```python
from build123d import *

# Parameters (mm, degrees)
BOSS_EXTRUDE1_OUTLINE_R = 5.250010824
BOSS_EXTRUDE1_DEPTH     = 19
CUT_EXTRUDE1_START      = -4
SKETCH2_R               = 8.500003527
CUT_EXTRUDE1_DEPTH      = 4
SKETCH3_R               = 8.500003527
CUT_EXTRUDE2_DEPTH      = 4
CUT_EXTRUDE3_START      = -4
CUT_EXTRUDE3_DEPTH      = 4
CUT_EXTRUDE4_DEPTH      = 4


# Read off the part's stored shape, not the designer's step: Boss-Extrude1
with BuildPart() as part:
    # Boss-Extrude1 outline → Boss-Extrude1 (new body)
    with BuildSketch(Plane.XY):
        with BuildLine():
            ThreePointArc((-23.133312794, -2.201771211), (-37.271533994, 6.292181292), (-28.786231545, -7.851233083))
            Line((-28.786231545, -7.851233083), (-26.586143602, -10.066323126))
            Line((-26.586143602, -10.066323126), (-26.23976909, -10.228203619))
            ThreePointArc((-26.23976909, -10.228203619), (-24.085157131, -11.906333766), (-21.354454149, -11.947983588))
            Line((-21.354454149, -11.947983588), (-10.14791118, -7.656975592))
            Line((-10.14791118, -7.656975592), (3.746314894, -9.374802435))
            Line((3.746314894, -9.374802435), (4.037513624, -7.019745673))
            Line((4.037513624, -7.019745673), (-11.498619188, -2.842881049))
            Line((-11.498619188, -2.842881049), (-20.193931688, -5.164955939))
            Line((-20.193931688, -5.164955939), (-23.133312794, -2.201771211))
        make_face()
        with Locations((-31.26296245, 0.27993313)):
            Circle(BOSS_EXTRUDE1_OUTLINE_R, mode=Mode.SUBTRACT)
    extrude(amount=BOSS_EXTRUDE1_DEPTH)

    # Sketch2 → Cut-Extrude1 (cut)
    with BuildSketch(Plane.XY.offset(19).offset(CUT_EXTRUDE1_START)):
        with Locations((-31.26296245, 0.27993313)):
            Circle(SKETCH2_R)
    extrude(amount=CUT_EXTRUDE1_DEPTH, mode=Mode.SUBTRACT)

    # Sketch3 → Cut-Extrude2 (cut)
    with BuildSketch(Plane(origin=(0, 0, 0), x_dir=(-1, 0, 0), z_dir=(0, 0, -1))):
        with Locations((31.26296245, 0.27993313)):
            Circle(SKETCH3_R)
    extrude(amount=-CUT_EXTRUDE2_DEPTH, mode=Mode.SUBTRACT)

    # Sketch4 → Cut-Extrude3 (cut)
    with BuildSketch(Plane.XY.offset(19).offset(CUT_EXTRUDE3_START)):
        with BuildLine():
            Line((-28.786231545, -7.851233083), (-27.3768314, -9.270243736))
            ThreePointArc((-27.3768314, -9.270243736), (-23.881833101, -7.115358231), (-21.724813867, -3.621676409))
            Line((-21.724813867, -3.621676409), (-23.133312794, -2.201771211))
            ThreePointArc((-23.133312794, -2.201771211), (-25.254390905, -5.732315031), (-28.786231545, -7.851233083))
        make_face()
    extrude(amount=CUT_EXTRUDE3_DEPTH, mode=Mode.SUBTRACT)

    # Sketch5 → Cut-Extrude4 (cut)
    with BuildSketch(Plane(origin=(0, 0, 0), x_dir=(-1, 0, 0), z_dir=(0, 0, -1))):
        with BuildLine():
            Line((23.133312794, -2.201771211), (21.719099232, -3.615984773))
            ThreePointArc((21.719099232, -3.615984773), (24.169813566, -6.821498289), (27.3768314, -9.270243736))
            Line((27.3768314, -9.270243736), (28.786231545, -7.851233083))
            ThreePointArc((28.786231545, -7.851233083), (25.254390905, -5.732315031), (23.133312794, -2.201771211))
        make_face()
    extrude(amount=-CUT_EXTRUDE4_DEPTH, mode=Mode.SUBTRACT)


solid = part.part
```
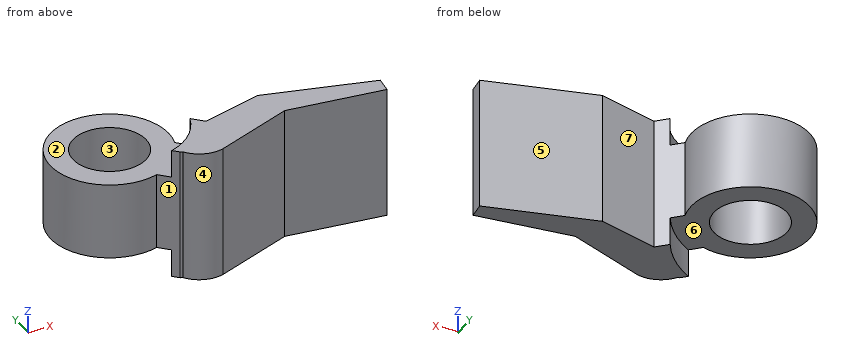
The listing builds one solid part. Answer for the finished solid, in the listing's coordinates (mm). Face numbers are marked on the shaded views. A direction names the side the tool comes from. Coordinates: 2 decimals unless noted, no trailing zeros. Order: outer loops, then holes, each group sorted by start corner. A loop starts at its lowest first (then second) coordinate and runs counter-clockwise, first axis right, second up. Notation, with made-up numbers: M 71,37.5 L 119,37.5 A8 cw 119,41.5 Z; hole C 56.5,3.25 d4. An arc over 180 degrees is marked long. Answer as a JSON object with one key per item and string values. Group by question number.
1. Flat-ended cylindrical pins translate along their axes: P1, Ø5.5, axis at x = -30, y = 1.5, coming from the +Z side; P2, Ø8, axis at x = -15, z = 10, coming from the +Y side; P3, Ø8, axis at x = -7, y = -4.5, coming from the -Z side; P4, Ø5, axis at y = 4, z = 9, coming from the +X side. Find the tip coordinate at first contact, or state that the pin passes through.
2. A tool of negligible diameter and unlimited length cuts with its end or side. For the marked faces 1, 2 and 3, from which of +Z, -Z, +X, -X, +Y, -Y can it reach the whole face along a straight path? Write none if from no direction.
3. Section A-A on x = -33.5 is taken. Write down the section's boundary in (y, z), then the cut area to 3 significant figures.
4. Section D-D on z = 10 is taken. Write down the section's boundary in (x, y).
5. Section B-B on z = 1.25 is taken. Write down the section's boundary in (x, y).
6. Straight lines are drawn through the part: line 1 (X direction, y = 0.5, z = 9.5); line 2 (X direction, y = 1.25, z = 13.25); line 3 (Z direction, x = -34.5, y = 4.5). For each, find the intervals that lie inside material, in ascending order.
7. Determine the mould class of the marked faces 4, 5, 6 and 7 for opening direction X: released by +X, released by -X, zero draft, split by the parting line, or undercut.
8. Section C-C on y = -1.5 is taken. Write down the section's boundary in (x, z).
Values follow:
{
 "1": {"P1": "through", "P2": "y = -2.84", "P3": "z = 0", "P4": "x = -22.85"},
 "2": {"face 1": "+Z, -Z, -Y", "face 2": "+Z, -X, +Y", "face 3": "+Z, -Z"},
 "3": {"outline": "M -7.92,4 L -4.47,4 L -4.47,15 L -7.92,15 Z; M 5.03,4 L 8.48,4 L 8.48,15 L 5.03,15 Z", "area": "75.9 mm2"},
 "4": {"outline": "M -28.79,-7.85 L -26.59,-10.07 L -26.24,-10.23 A4.3 ccw -21.35,-11.95 L -10.15,-7.66 L 3.75,-9.37 L 4.04,-7.02 L -11.5,-2.84 L -20.19,-5.16 L -23.13,-2.2 A8.5 ccw long Z; hole C -31.26,0.28 d10.5"},
 "5": {"outline": "M -27.38,-9.27 L -26.59,-10.07 L -26.24,-10.23 A4.3 ccw -21.35,-11.95 L -10.15,-7.66 L 3.75,-9.37 L 4.04,-7.02 L -11.5,-2.84 L -20.19,-5.16 L -21.72,-3.62 A15.22 cw Z"},
 "6": {"line 1": "-39.76 to -36.51, -26.02 to -22.77", "line 2": "-39.71 to -36.42, -26.1 to -22.82", "line 3": "4 to 15"},
 "7": {"face 4": "split by the parting line", "face 5": "released by +X", "face 6": "zero draft", "face 7": "undercut"},
 "8": {"outline": "M -39.57,4 L -36.2,4 L -36.2,15 L -39.57,15 Z; M -26.32,4 L -22.95,4 L -22.95,15 L -26.32,15 Z"}
}
